Can you work these out from the model? Positions are in its coordinate system, mm. Face numbers are marked on the shaded views. A direction names the side the tool comes from. Coordinates: 2 decimals unless noted, no trailing zeros. Write each loop counter-clockwise with the first axis right and the second up, starting at its lowest first coordinate (ties: lowest second). Pieces come first, ordered by that corner, then holes.
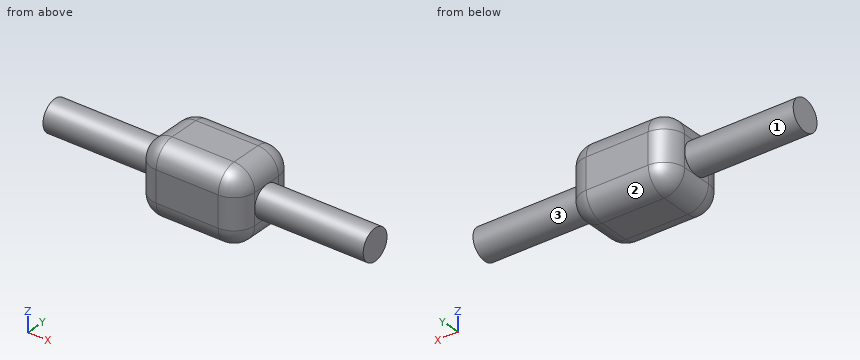
```python
from build123d import *

# Parameters (mm, degrees)
SKETCH_2_R      = 7.5
EXTRUDE_1_DEPTH = 77.5
SKETCH_3_W      = 35
SKETCH_3_H      = 35
EXTRUDE_2_DEPTH = 25
FILLET_1_R      = 10
FILLET_2_R      = 10


with BuildPart() as part:
    # 草图2 → 凸台-拉伸1 (new, symmetric)
    with BuildSketch(Plane(origin=(0, 0, 0), x_dir=(0, 0, -1), z_dir=(1, 0, 0))):
        Circle(SKETCH_2_R)
    extrude(amount=EXTRUDE_1_DEPTH, both=True)

    # 草图3 → 凸台-拉伸2 (add, symmetric)
    with BuildSketch(Plane(origin=(0, 0, 0), x_dir=(0, 0, -1), z_dir=(1, 0, 0))):
        Rectangle(SKETCH_3_W, SKETCH_3_H)
    extrude(amount=EXTRUDE_2_DEPTH, both=True)

    # 圆角1
    fillet_1_edges = [part.edges().sort_by_distance(p)[0] for p in [
        (0, 17.5, 17.5),
        (0, -17.5, 17.5),
        (0, -17.5, -17.5),
        (0, 17.5, -17.5),
    ]]
    fillet(fillet_1_edges, radius=FILLET_1_R)

    # 圆角2
    fillet_2_edges = [part.edges().sort_by_distance(p)[0] for p in [
        (-25, 0, -17.5),
        (25, 0, -17.5),
        (-25, 0, 17.5),
        (-25, 17.5, 0),
        (-25, -17.5, 0),
        (-25, 14.571067812, 14.571067812),
        (-25, -14.571067812, 14.571067812),
        (-25, 14.571067812, -14.571067812),
        (-25, -14.571067812, -14.571067812),
        (25, -17.5, 0),
        (25, 0, 17.5),
        (25, 17.5, 0),
        (25, 14.571067812, 14.571067812),
        (25, -14.571067812, 14.571067812),
        (25, 14.571067812, -14.571067812),
        (25, -14.571067812, -14.571067812),
    ]]
    fillet(fillet_2_edges, radius=FILLET_2_R - 0.0001)  # a hair under: the kernel refuses the full size


solid = part.part
```
1. If we section it at D-D, the plane x = -40: List the corners of the cut face in (y, z) for me, plus the area to 3 significant figures.
2. If we section it at C-C, the plane x = -3: List the corners of the cut face in (y, z) for me, plus the area to 3 significant figures.
3. I'm going to push flat-ended pins straight in: P1, Ø1.5, axis at y = -12.5, z = -13.5, coming from the -X side; P2, Ø8, axis at x = -54, z = -5.5, coming from the -Y side; P3, Ø5, axis at y = -9, z = 13.5, coming from the +X side. Where does each tip first touch, or does it pass through?
4. If I drill on L1, parallel to X at y = -2.5, z = -7.5; L2, parallel to X at y = 11, z = 12; L3, parallel to Z at x = 0, y = 9, over which ranges is the centre line in solid material (lowest first)?
5. Which directions (+Z, -Z, +X, -X, +Y, -Y) give clear straight access to the entire face, cutting with the end or side of a thin tool? Please do the marked faces 1, 2 and 3.
Answers:
1. outline: circle Ø15 at (0, 0)
1. area: 177 mm2
2. outline: (-17.5, -7.5) arc R10 ccw to (-7.5, -17.5) - (7.5, -17.5) arc R10 ccw to (17.5, -7.5) - (17.5, 7.5) arc R10 ccw to (7.5, 17.5) - (-7.5, 17.5) arc R10 ccw to (-17.5, 7.5) - close
2. area: 1,140 mm2
3. P1: stops at x = -22.08
3. P2: stops at y = -7.35
3. P3: stops at x = 24.3
4. L1: x = -25 to 25
4. L2: x = -23.22 to 23.22
4. L3: z = -17.39 to 17.39
5. face 1: -X
5. face 2: -Z, +X, -X, +Y
5. face 3: +X
